Input: part model. Units: mm. Frame: model coordinates. Give positions to 0.01 mm unless a question says otherwise; leave off trailing zeros. Write each loop counter-clockwise with the first axis right and the second up, starting at its lowest first coordinate (ties: lowest second). Pieces come first, ordered by that corner, then holes. Notation, with made-up numbers: (7.25, -2) - (12.25, -2) arc R33 cw to (12.25, 29) - close; hole circle Ø7 at (54.25, 8.25). An arc over 180 degrees is marked (long way). Answer as CSV lines item,"result". Start each with the question number.
from build123d import *

# Parameters (mm, degrees)
SKETCH_1_W          = 506
SKETCH_1_H          = 72
SKETCH_1_R          = 25
SKETCH_1_R_2        = 2.75
EXTRUDE_1_DEPTH     = 5
CHAMFER_1_SIZE      = 5
SKETCH_2_R          = 2.5
CUT_EXTRUDE_1_DEPTH = 256.597339579


with BuildPart() as part:
    # 草图1 → 凸台-拉伸1 (new body)
    with BuildSketch(Plane.XY):
        Rectangle(SKETCH_1_W, SKETCH_1_H)
        with Locations((223, 0)):
            Circle(SKETCH_1_R, mode=Mode.SUBTRACT)
        with Locations((247.748737342, 24.748737342)):
            Circle(SKETCH_1_R_2, mode=Mode.SUBTRACT)
        with Locations((198.251262658, 24.748737342)):
            Circle(SKETCH_1_R_2, mode=Mode.SUBTRACT)
        with Locations((198.251262658, -24.748737342)):
            Circle(SKETCH_1_R_2, mode=Mode.SUBTRACT)
        with Locations((247.748737342, -24.748737342)):
            Circle(SKETCH_1_R_2, mode=Mode.SUBTRACT)
        with Locations(Location((-247.748737342, -24.748737342, 0), (0, 0, 180))):
            Circle(SKETCH_1_R_2, mode=Mode.SUBTRACT)
        with Locations(Location((-247.748737342, 24.748737342, 0), (0, 0, 180))):
            Circle(SKETCH_1_R_2, mode=Mode.SUBTRACT)
        with Locations(Location((-198.251262658, 24.748737342, 0), (0, 0, 180))):
            Circle(SKETCH_1_R_2, mode=Mode.SUBTRACT)
        with Locations(Location((-198.251262658, -24.748737342, 0), (0, 0, 180))):
            Circle(SKETCH_1_R_2, mode=Mode.SUBTRACT)
        with Locations(Location((-223, 0, 0), (0, 0, 180))):
            Circle(SKETCH_1_R, mode=Mode.SUBTRACT)
    extrude(amount=EXTRUDE_1_DEPTH)

    # 倒角1
    chamfer_1_edges = [part.edges().sort_by_distance(p)[0] for p in [
        (-253, 36, 2.5),
        (253, 36, 2.5),
        (253, -36, 2.5),
        (-253, -36, 2.5),
    ]]
    chamfer(chamfer_1_edges, length=CHAMFER_1_SIZE)

    # 草图2 → 切除-拉伸1 (cut, through all)
    with BuildSketch(Plane.XY.offset(5)):
        with Locations((-122, 26)):
            Circle(SKETCH_2_R)
        with Locations((-122, -26)):
            Circle(SKETCH_2_R)
        with Locations((-106, 26)):
            Circle(SKETCH_2_R)
        with Locations((-106, -26)):
            Circle(SKETCH_2_R)
        with Locations(Location((106, -26, 0), (0, 0, 180))):
            Circle(SKETCH_2_R)
        with Locations(Location((106, 26, 0), (0, 0, 180))):
            Circle(SKETCH_2_R)
        with Locations(Location((122, -26, 0), (0, 0, 180))):
            Circle(SKETCH_2_R)
        with Locations(Location((122, 26, 0), (0, 0, 180))):
            Circle(SKETCH_2_R)
    extrude(amount=-CUT_EXTRUDE_1_DEPTH, mode=Mode.SUBTRACT)


solid = part.part
1) Cut plane B-B on y = -12.5. Output: boundary loops of the cut face in (x, z), and give its area (3 significant figures).
2) Cut plane C-C on z = 2.75. State how many separate pieces and enclosed holes the cut face has, and give its area (3 significant figures).
3) Material intervals for line 1 (Y direction, x = -122, z = 2.2); line 2 (X direction, y = -11.5, z = 4.5); line 3 (X direction, y = 6.5, z = 0.6), sorted ascending. Write a range as from..to.
4) Cut plane D-D on y = 16. Output: boundary loops of the cut face in (x, z).
5) Cut plane A-A on x = -223. Output: boundary loops of the cut face in (y, z).
6) Pull-direction query (Y, two-part tool) for faces 1 (the cylindrical face through (246.846, 7.509, 2.465)), 2 (the flat face through (-4, 1, 5)), 3 (the cylindrical face through (-246.846, -7.509, 2.465)); classes: +Y half, -Y half, draft (parallel to the pull), parting line (faces both ways), or undercut.
Numbers:
1,outline,"(-253, 0) - (-244.65, 0) - (-244.65, 5) - (-253, 5) - close; (-201.35, 0) - (201.35, 0) - (201.35, 5) - (-201.35, 5) - close; (244.65, 0) - (253, 0) - (253, 5) - (244.65, 5) - close"
1,area,"2,100 mm²"
2,separate pieces,"1"
2,enclosed holes,"18"
2,area,"32,100 mm²"
3,line 1,"y = -36..-28.5, -23.5..23.5, 28.5..36"
3,line 2,"x = -253..-245.2, -200.8..200.8, 245.2..253"
3,line 3,"x = -253..-247.14, -198.86..198.86, 247.14..253"
4,outline,"(-253, 0) - (-242.21, 0) - (-242.21, 5) - (-253, 5) - close; (-203.79, 0) - (203.79, 0) - (203.79, 5) - (-203.79, 5) - close; (242.21, 0) - (253, 0) - (253, 5) - (242.21, 5) - close"
5,outline,"(-36, 0) - (-25, 0) - (-25, 5) - (-36, 5) - close; (25, 0) - (36, 0) - (36, 5) - (25, 5) - close"
6,face 1,"undercut"
6,face 2,"draft"
6,face 3,"undercut"
